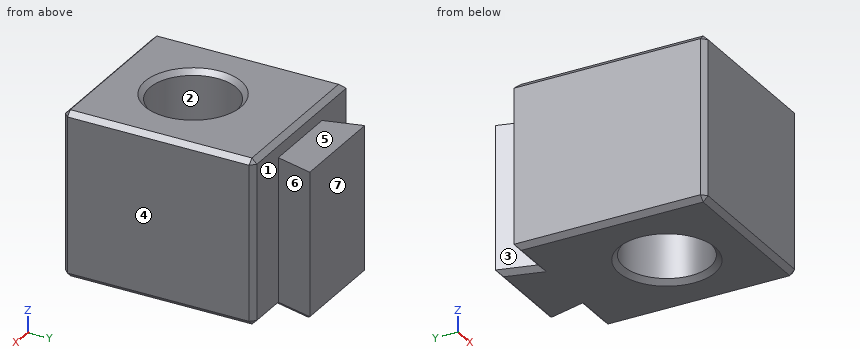
```python
from build123d import *

# Parameters (mm, degrees)
F2_R     = 5.25
F3_DEPTH = 20
F4_DEPTH = 18
F5_SIZE  = 0.6


# Not quite as in the source:
# - a feature names something its author has since deleted; it is built from what else it names


with BuildPart() as f3:
    # F2 (on Top) → F3 (new body)
    with BuildSketch(Plane.XY):
        Polygon((5.25, 23.25), (0, 23.25), (0, 0), (20, 0), (20, 23.25), (14.75, 23.25), align=None)
        with Locations((10, 10.25)):
            Circle(F2_R, mode=Mode.SUBTRACT)
    extrude(amount=F3_DEPTH)

    # F2 (on Top) → F4 (join)
    with BuildSketch(Plane.XY):
        Polygon((4.0442286341, 27.75), (5.25, 23.25), (14.75, 23.25), (15.9557713659, 27.75), align=None)
    extrude(amount=F4_DEPTH)

    # F5
    f5_edges = [f3.edges().sort_by_distance(p)[0] for p in [
        (0, 11.625, 0),
        (10, 0, 0),
        (20, 11.625, 0),
        (17.375, 23.25, 0),
        (15.352886, 25.5, 0),
        (10, 27.75, 0),
        (4.647114, 25.5, 0),
        (2.625, 23.25, 0),
        (4.75, 10.25, 0),
        (10, 23.25, 20),
        (0, 11.625, 20),
        (10, 0, 20),
        (20, 11.625, 20),
        (4.75, 10.25, 20),
        (0, 0, 10),
        (20, 0, 10),
        (20, 23.25, 10),
    ]]
    chamfer(f5_edges, length=F5_SIZE)


solid = f3.part
```
Can you work these out from the model? Positions are in its coordinate system, mm. Face numbers are marked on the shaded views. A direction names the side the tool comes from. Give positions to 0.01 mm unless a question says otherwise; leave off trailing zeros. Order: outer loops, then holes, each group sorted by start corner. A loop starts at its lowest first (then second) coordinate and runs counter-clockwise, first axis right, second up. Notation, with made-up numbers: (66.5, 87.25) - (101.5, 87.25) arc R21 ccw to (101.5, 111.25) - close; hole circle Ø7 at (20, 32.25). An arc over 180 degrees is marked (long way). Use a Markdown table: item, result. Add a question column.
Q1. I'm going to push flat-ended pins straight in: pin 1 (1 mm diameter, centred on x = 4.5, y = 10.5, fed in from -Z); pin 2 (3 mm diameter, centred on x = 13, y = 7.5, fed in from -Z); pin 3 (8.5 mm diameter, centred on x = 10, y = 10.25, fed in from +Z); pin 4 (2 mm diameter, centred on x = 9, y = 26.5, fed in from +Z). Where does each tip first touch, or does it pass through?
Q2. On a 3-axis mill with a long thin cutter (end or side, diameter ignored), from which of +Z, -Z, +X, -X, +Y, -Y can I reach the whole of each face in a straight line? I mean the marked faces 5, 6 and 7. Say none if no direction works.
Q3. If we section it at A-A on y = 10.25: Write out the boundary of the cut face in (x, z), plus the area to 3 significant figures.
Q4. If we section it at B-B on x = 10: Write out the boundary of the cut face in (y, z).
Q5. If we section it at D-D on x = 17.75: Write out the boundary of the cut face in (y, z), plus the area to 3 significant figures.
Q6. Please list where these lines run through material, in increasing order: line 1 along Y through (x, z) = (10, 7.5); line 2 along X through (y, z) = (12.5, 8); line 3 along Y through (x, z) = (6, 14.75).
Q7. If we section it at C-C on z = 13: Write out the boundary of the cut face in (x, y).
Q8. If we mould it in two halves opening along X, with no side actions, what happens to the marked faces 1, 2, 3 and 4? For each: released by +X, released by -X, zero draft, split by the parting line, or undercut.
Answers follow:
| question | item | result |
|---|---|---|
| 1 | pin 1 | stops at z = 0 |
| 1 | pin 2 | stops at z = 0.28 |
| 1 | pin 3 | passes through |
| 1 | pin 4 | stops at z = 18 |
| 2 | face 5 | +Z, +X, -X, +Y |
| 2 | face 6 | +Z, -Z, +X |
| 2 | face 7 | +Z, -Z, +X, -X, +Y |
| 3 | outline | (0, 0.6) - (0.6, 0) - (4.15, 0) - (4.75, 0.6) - (4.75, 19.4) - (4.15, 20) - (0.6, 20) - (0, 19.4) - close; (15.25, 0.6) - (15.85, 0) - (19.4, 0) - (20, 0.6) - (20, 19.4) - (19.4, 20) - (15.85, 20) - (15.25, 19.4) - close |
| 3 | area | 189 mm^2 |
| 4 | outline | (0, 0.6) - (0.6, 0) - (4.4, 0) - (5, 0.6) - (5, 19.4) - (4.4, 20) - (0.6, 20) - (0, 19.4) - close; (15.5, 0.6) - (16.1, 0) - (27.15, 0) - (27.75, 0.6) - (27.75, 18) - (23.25, 18) - (23.25, 19.4) - (22.65, 20) - (16.1, 20) - (15.5, 19.4) - close |
| 5 | outline | (0, 0.6) - (0.6, 0) - (22.65, 0) - (23.25, 0.6) - (23.25, 19.4) - (22.65, 20) - (0.6, 20) - (0, 19.4) - close |
| 5 | area | 464 mm^2 |
| 6 | line 1 | y = 0 to 5, 15.5 to 27.75 |
| 6 | line 2 | x = 0 to 5.26, 14.74 to 20 |
| 6 | line 3 | y = 0 to 6.85, 13.65 to 27.75 |
| 7 | outline | (0, 0.6) - (0.6, 0) - (19.4, 0) - (20, 0.6) - (20, 22.65) - (19.4, 23.25) - (14.75, 23.25) - (15.96, 27.75) - (4.04, 27.75) - (5.25, 23.25) - (0, 23.25) - close; hole circle Ø10.5 at (10, 10.25) |
| 8 | face 1 | zero draft |
| 8 | face 2 | undercut |
| 8 | face 3 | released by -X |
| 8 | face 4 | released by +X |
